Read the model definition and answer for the solid it produces. Units are mm, in the model's axes. A direction names the side the tool comes from. Round coordinates to 2 decimals unless told otherwise and drop trailing zeros. Order: outer loops, then holes, each group sorted by start corner. A loop starts at its lowest first (then second) coordinate and runs counter-clockwise, first axis right, second up.
Autodesk Inventor part; units mm, degrees
ref_plane "YZ Plane" through (0, 0, 0) normal (1, 0, 0) x (0, 1, 0)
ref_plane "XZ Plane" through (0, 0, 0) normal (0, 1, 0) x (-1, 0, 0)
ref_plane "XY Plane" through (0, 0, 0) normal (0, 0, 1) x (1, 0, 0)
sketch "Boceto1" plane through (0, 0, 0) normal (1, 0, 0) x (0, 1, 0)
  line L0 (0, 0) -> (0, -3)
  line L1 (0, -3) -> (10, -3)
  line L2 (10, -3) -> (10, 0)
  line L3 (10, 0) -> (20, 0)
  line L4 (20, 0) -> (20, -3)
  line L5 (20, -3) -> (30, -3)
  line L6 (30, -33.4269) -> (30, -40)
  line L7 (30, -40) -> (20, -40)
  line L8 (20, -40) -> (20, -43)
  line L9 (20, -43) -> (10, -43)
  line L10 (10, -43) -> (10, -40)
  line L11 (10, -40) -> (0, -40)
  circle A0 centre (15, -21.5) radius 13.175
  arc A1 (0, -9.5731) -> (0, -33.4269) centre (15, -21.5) ccw
  arc A2 (30, -33.4269) -> (30, -9.5731) centre (15, -21.5) ccw
  line L12 (0, -40) -> (0, -33.4269)
  line L13 (0, -9.5731) -> (0, -3)
  line L14 (30, -3) -> (30, -9.5731)
  dimension "d1" = 10
  dimension "d2" = 10
  dimension "d3" = 10
extrude "Extrusión1" add sketch "Boceto1" along normal blind 3
sketch "Boceto2" plane through (3, 0, 0) normal (1, 0, 0) x (0, 0, -1)
  line L0 (3, 10) -> (3, 0)
  line L1 (3, 0) -> (0, 0)
  line L2 (0, 20) -> (0, 10)
  line L3 (0, 0) -> (0, 10)
  line L4 (0, 10) -> (-3, 10)
  line L5 (-3, 10) -> (-3, 20)
  line L6 (-3, 20) -> (0, 20)
  line L7 (0, 20) -> (0, 30)
  line L8 (3, 30) -> (3, 20)
  line L9 (0, 30) -> (3, 30)
  line L10 (3, 30) -> (3, 20)
  line L11 (3, 20) -> (0, 20)
  line L12 (3, 20) -> (0, 20)
  line L13 (0, 20) -> (0, 10)
  line L14 (0, 10) -> (3, 10)
  line L15 (3, 0) -> (3, 10)
  dimension "d11" = 3
extrude "Extrusión2" add sketch "Boceto2" against normal blind 3
properties part number "cod"
Q1. Straight lines are drawn through the part: probe 1 along Z at (x, y) = (0.9, 15) (3 decimals); probe 2 along Y at (x, z) = (2, -7); probe 3 along Z at (x, y) = (0.3, 9). For each, find the intervals that lie inside material, in ascending order.
Outcome:
probe 1: z = -43 to -34.675, -8.325 to 3
probe 2: y = 0 to 30
probe 3: z = -40 to -33.23, -9.77 to 0
Q2. A cutting plane is placed at B-B, the plane z = -21.5. Give the vertices of the cut face in (x, y) (3 decimals), plus the area to 3 significant figures.
Outcome:
outline: (0, -4.164) - (3, -4.164) - (3, 1.825) - (0, 1.825) - close; (0, 28.175) - (3, 28.175) - (3, 34.164) - (0, 34.164) - close
area: 35.9 mm2
Q3. For faces 4 (the face through (1, 20, -41)), 5 (the face through (2, 20, 2)), 6 (the face through (2, 15, 3)), 7 (the face through (1, 5, -40)), 8 (the face through (2, 5, 0)), determine the directions among +Z, -Z, +X, -X, +Y, -Y from which every point of the face is accessible in a straight line to the end or side of a thin tool.
Outcome:
face 4: -Z, +X, -X, +Y
face 5: +Z, +X, -X, +Y
face 6: +Z, +X, -X, +Y, -Y
face 7: -Z, +X, -X, -Y
face 8: +Z, +X, -X, -Y
Q4. Flat-ended cylindrical pins translate along their axes: pin 1 (1.5 mm diameter, centred on x = 2, y = 5, fed in from -Z); pin 2 (1.5 mm diameter, centred on x = 1, z = -41, fed in from -Y); pin 3 (0.9 mm diameter, centred on x = 1.5, z = -41, fed in from +Y). Find the tip coordinate at first contact, or state that the pin passes through.
Outcome:
pin 1: stops at z = -40
pin 2: stops at y = 10
pin 3: stops at y = 20
Q5. For a pull along Z with two mould halves and no side action, classify faces 1 (the face through (1.48, 21.08, -9.81)), 2 (the face through (1.479, -4.163, -21.68)), 3 (the face through (1, 15, -43)) as released by +Z, released by -Z, zero draft, split by the parting line, or undercut.
Outcome:
face 1: undercut
face 2: split by the parting line
face 3: released by -Z
Q6. A cutting plane is placed at D-D, the plane z = -2. Give the vertices of the cut face in (x, y).
Outcome:
outline: (0, 0) - (3, 0) - (3, 30) - (0, 30) - close
Q7. A cutting plane is placed at C-C, the plane x = 0.7. Give the vertices of the cut face in (y, z) (3 decimals).
Outcome:
outline: (0, -40) - (10, -40) - (10, -43) - (20, -43) - (20, -40) - (30, -40) - (30, -33.427) arc R19.164 ccw to (30, -9.573) - (30, 0) - (20, 0) - (20, 3) - (10, 3) - (10, 0) - (0, 0) - (0, -9.573) arc R19.164 ccw to (0, -33.427) - close; hole circle Ø26.35 at (15, -21.5)
Q8. A cutting plane is placed at A-A, the plane y = 15. Give the vertices of the cut face in (x, z) (3 decimals).
Outcome:
outline: (0, -43) - (3, -43) - (3, -34.675) - (0, -34.675) - close; (0, -8.325) - (3, -8.325) - (3, 3) - (0, 3) - close
